Work out the finished part from the listing and answer in its coordinate system (mm). Face numbers are marked on the shaded views. Give positions to 0.01 mm unless a question says otherwise; leave off trailing zeros. Loops run counter-clockwise (first coordinate to the right, second up) from the corner with the lowest first, then second, coordinate; pieces in that order, holes last. Notation, with made-up numbers: M 69,42.25 L 81,42.25 A23 cw 81,74.25 Z; hole C -26.75,76.25 d7. An arc over 180 degrees is marked long. Answer as a JSON object with one key per item and string values. Group by question number.
```python
from build123d import *

# Parameters (mm, degrees)
BASE_FLANGE1_DEPTH = 10


# Sheet-metal steps are written as plain solids
with BuildPart() as part:
    # Sketch2 → Base-Flange1 (new body)
    with BuildSketch(Plane(origin=(0, 0, 0), x_dir=(1, 0, 0), z_dir=(0, 1, 0))):
        with BuildLine():
            ThreePointArc((11.5, -4.898979486), (-12.247448714, 2.5), (12.5, 0))
            Line((12.5, 0), (12.5, -20))
            Line((12.5, -20), (11.7, -20))
            Line((11.7, -20), (11.7, 0))
            ThreePointArc((11.7, 0), (-11.463611996, 2.34), (10.764, -4.585444798))
            Line((10.764, -4.585444798), (11.5, -4.898979486))
        make_face()
    extrude(amount=BASE_FLANGE1_DEPTH)


solid = part.part
```
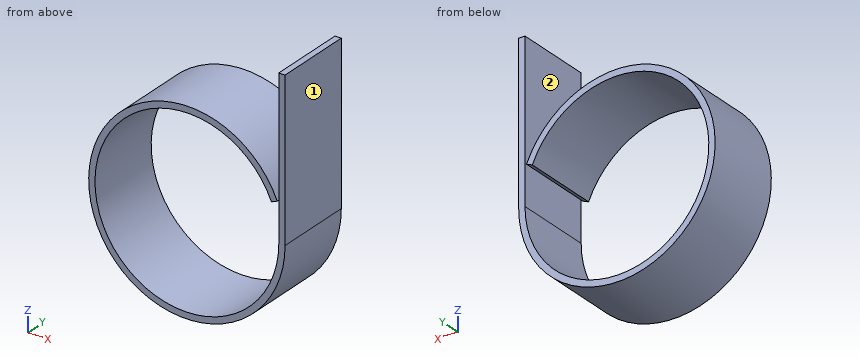
Item 1: Given pin 1 Ø2 at (x, z) = (-0.5, -9) entering from -Y; pin 2 Ø4 at (y, z) = (2, -5.5) entering from -X; pin 3 Ø2 at (x, y) = (9.5, 3.5) entering from -Z; pin 4 Ø6 at (x, y) = (4, 7) entering from +Z, each flat-ended and moving along its own axis, determine where each tip first touches the part or whether it passes through.
Item 2: Find the intervals of material crossed by probe 1 along X at (y, z) = (3.5, 0); probe 2 along X at (y, z) = (6, 7.5), in increasing order. Write a range as [from, to].
Item 3: A cutting plane is placed at D-D (z = 6). Determine the outline of the cut face in (x, y).
Item 4: A cutting plane is placed at B-B (z = 2.5). Determine the outline of the cut face in (x, y).
Item 5: A cutting plane is placed at A-A (x = 0). Determine the outline of the cut face in (y, z), and give its area (3 significant figures).
Item 6: A cutting plane is placed at C-C (y = 5.25). Determine the outline of the cut face in (x, z), and give its area (3 significant figures).
Item 7: For a pull along X with two mould halves and no side action, classify the marked faces 1 and 2 as pulls with the +X half, pulls with the -X half, needs draft (parallel to the pull), parting line crosses it, or undercut.
The answers:
{
 "1": {"pin 1": "passes through", "pin 2": "stops at x = -12", "pin 3": "stops at z = -9.17", "pin 4": "stops at z = 12.46"},
 "2": {"probe 1": "x = [-12.5, -11.7], [11.7, 12.5]", "probe 2": "x = [-10, -8.98], [8.98, 10], [11.7, 12.5]"},
 "3": {"outline": "M -10.97,0 L -10.04,0 L -10.04,10 L -10.97,10 Z; M 10.04,0 L 10.97,0 L 10.97,10 L 10.04,10 Z; M 11.7,0 L 12.5,0 L 12.5,10 L 11.7,10 Z"},
 "4": {"outline": "M -12.25,0 L -11.43,0 L -11.43,10 L -12.25,10 Z; M 11.7,0 L 12.5,0 L 12.5,10 L 11.7,10 Z"},
 "5": {"outline": "M 0,-12.5 L 10,-12.5 L 10,-11.7 L 0,-11.7 Z; M 0,11.7 L 10,11.7 L 10,12.5 L 0,12.5 Z", "area": "16.0 mm^2"},
 "6": {"outline": "M 10.76,4.59 L 11.5,4.9 A12.5 ccw long 12.5,0 L 12.5,20 L 11.7,20 L 11.7,0 A11.7 cw long Z", "area": "72.9 mm^2"},
 "7": {"face 1": "pulls with the +X half", "face 2": "undercut"}
}
